Autodesk Inventor part; units mm, degrees
ref_plane "Work Plane3" through (-47.3429, 25.922, -109.9566) normal (0, 1, 0) x (1, 0, 0)
ref_plane "Work Plane4" through (-11.7245, 25.1265, -109.9566) normal (0, -1, 0) x (-1, 0, 0)
ref_plane "YZ Plane" through (0, 0, 0) normal (1, 0, 0) x (0, 1, 0)
sketch "Sketch1" plane through (0, 0, 0) normal (0, 0, 1) x (1, 0, 0)
  point P0 (0, 0)
sketch "Sketch2" plane through (0, 0, 0) normal (0, 1, 0) x (-1, 0, 0)
  line L0 (29.4419, 0) -> (29.4988, 0)
  arc A0 (58.9407, -29.4419) -> (29.4988, 0) centre (29.4988, -29.4419) ccw
  arc A1 (29.4419, 0) -> (0, -29.4419) centre (29.4419, -29.4419) ccw
  line L1 (0, -29.4419) -> (1.3334, -33.4091)
  line L2 (1.3334, -33.4091) -> (1.3334, -74.6587)
  line L3 (1.3334, -74.6587) -> (0, -77.6285)
  line L4 (0, -77.6285) -> (-1.0327, -97.9222)
  line L5 (58.9407, -29.4419) -> (57.7766, -33.4091)
  line L6 (57.7766, -33.4091) -> (57.7766, -76.7951)
  line L7 (57.7766, -76.7951) -> (58.9407, -78.9752)
  line L8 (58.9407, -78.9752) -> (59.9743, -95.7523)
  line L9 (59.9743, -95.7523) -> (60.0189, -96.4757)
  line L10 (-1.0327, -97.9222) -> (-0.9556, -96.5463)
  line L11 (11.7245, -109.9566) -> (47.3429, -109.9566)
  arc A2 (47.3429, -109.9566) -> (60.0189, -96.4757) centre (47.3429, -97.2566) ccw
  arc A3 (-0.9556, -96.5463) -> (11.7245, -109.9566) centre (11.7245, -97.2566) ccw
  point P0 (0, 0)
  point P1 (58.9407, 0)
  dimension "d5" = 29.4419
  dimension "d6" = 41.2496
  dimension "d7" = 20.32
  dimension "d8" = 12.7
extrude "Extrusion1" add sketch "Sketch2" along normal blind 29.5148
sketch "Sketch3" plane through (0, 29.5148, 0) normal (0, 1, 0) x (1, 0, 0)
  line L0 (-29.7463, 1.6533) -> (-29.8195, 1.6533)
  arc A0 (-58.3691, 30.2029) -> (-29.8195, 1.6533) centre (-29.8195, 30.2029) ccw
  arc A1 (-29.7463, 1.6533) -> (-1.1967, 30.2029) centre (-29.7463, 30.2029) ccw
  line L1 (-1.1967, 30.2029) -> (-2.4901, 33.4321)
  line L2 (-2.4901, 33.4321) -> (-2.4901, 73.4442)
  line L3 (-2.4901, 73.4442) -> (-0.5766, 76.9439)
  line L4 (-0.5766, 76.9439) -> (0.4251, 96.6289)
  line L5 (-58.3691, 30.2029) -> (-56.62, 33.4321)
  line L6 (-56.62, 33.4321) -> (-56.62, 75.5165)
  line L7 (-56.62, 75.5165) -> (-57.7491, 78.2503)
  line L8 (-57.7491, 78.2503) -> (-58.7517, 94.5241)
  line L9 (-58.7517, 94.5241) -> (-58.7949, 95.2257)
  line L10 (0.4251, 96.6289) -> (0.3503, 95.2942)
  line L11 (-11.9494, 108.3022) -> (-46.4992, 108.3022)
  arc A2 (-46.4992, 108.3022) -> (-58.7949, 95.2257) centre (-46.4992, 95.9832) ccw
  arc A3 (0.3503, 95.2942) -> (-11.9494, 108.3022) centre (-11.9494, 95.9832) ccw
  line L12 (-2.4901, 52.1447) -> (-2.4901, 53.4382) construction
  line L13 (-57.7766, 76.7951) -> (-57.7766, 33.4091) construction
  line L14 (-57.7766, 54.1324) -> (-56.62, 54.1324) construction
  arc A4 (-58.9407, 29.4419) -> (-29.4988, 0) centre (-29.4988, 29.4419) ccw construction
  line L15 (-29.4988, 0) -> (-29.4988, 1.6544) construction
  line L16 (-28.1015, 108.3022) -> (-28.1015, 109.9566) construction
  line L17 (-11.7245, 109.9566) -> (-47.3429, 109.9566) construction
  line L18 (-2.4901, 53.4382) -> (-1.3334, 53.4382) construction
  line L19 (-1.3334, 33.4091) -> (-1.3334, 74.6587) construction
  point P0 (0, 0)
  point P1 (-1.2057, 1.6533)
  point P2 (-58.3782, 1.6533)
  dimension "d9" = 28.5496
  dimension "d10" = 40.0121
  dimension "d11" = 19.7104
  dimension "d12" = 12.319
extrude "Extrusion2" cut sketch "Sketch3" against normal blind 25.4
sketch "Sketch4" plane through (0, 29.5148, 0) normal (0, 1, 0) x (1, 0, 0)
  point P0 (0, 0)
sketch "Sketch5" plane through (-11.7245, 0, -109.9566) normal (0, 0, -1) x (-1, 0, 0)
  line L0 (35.6184, 26.9603) -> (35.6184, 25.922)
  line L1 (35.6184, 0) -> (35.6184, 29.5148)
  line L2 (0, 0) -> (0, 29.5148)
  point P0 (-11.7245, 0)
sketch "Sketch6" plane through (0, 29.5148, 0) normal (0, 1, 0) x (1, 0, 0)
  point P0 (0, 0)
ref_plane "Work Plane3" through (-47.3429, 25.922, -109.9566) normal (0, 1, 0) x (1, 0, 0)
sketch "Sketch7" plane through (-47.3429, 25.922, -109.9566) normal (0, 1, 0) x (1, 0, 0)
  line L0 (46.0094, -76.5475) -> (46.0094, -35.2979)
  line L1 (46.0094, -35.2979) -> (47.3429, -32.3281)
  line L2 (47.3429, -32.3281) -> (48.2985, -13.4103)
  line L3 (48.2985, -13.4103) -> (48.3756, -12.0344)
  line L4 (46.0094, -76.5475) -> (47.3429, -80.5147)
  line L5 (0, 0) -> (35.6184, 0)
  line L6 (-12.676, -13.4809) -> (-11.5978, -30.9814)
  line L7 (-11.5978, -30.9814) -> (-10.4337, -33.1615)
  line L8 (-10.4337, -33.1615) -> (-10.4337, -76.5475)
  line L9 (-10.4337, -76.5475) -> (-11.5978, -80.5147)
  arc A0 (-11.5978, -80.5147) -> (47.3429, -80.5147) centre (17.8725, -80.5147) ccw
  arc A1 (48.3756, -12.0344) -> (35.6184, 0) centre (35.6184, -12.7789) ccw
  line L10 (-12.676, -13.4809) -> (-11.5978, -30.9814)
  arc A2 (0, 0) -> (-12.676, -13.4809) centre (0, -12.7) ccw
  line L11 (46.0094, -76.5475) -> (46.0094, -35.2979)
  line L12 (46.0094, -35.2979) -> (47.3429, -32.3281)
  line L13 (47.3429, -32.3281) -> (48.2985, -13.4103)
  line L14 (48.2985, -13.4103) -> (48.3756, -12.0344)
  line L15 (46.0094, -76.5475) -> (47.3429, -80.5147)
  line L16 (0, 0) -> (35.6184, 0)
  line L17 (-12.676, -13.4809) -> (-11.5978, -30.9814)
  line L18 (-11.5978, -30.9814) -> (-10.4337, -33.1615)
  line L19 (-10.4337, -33.1615) -> (-10.4337, -76.5475)
  line L20 (-10.4337, -76.5475) -> (-11.5978, -80.5147)
  arc A3 (-11.5978, -80.5147) -> (47.3429, -80.5147) centre (17.8725, -80.5147) ccw
  arc A4 (48.3756, -12.0344) -> (35.6184, 0) centre (35.6184, -12.7789) ccw
  arc A5 (0, 0) -> (-12.676, -13.4809) centre (0, -12.7) ccw
  point P0 (47.3429, -109.9566)
sketch "Sketch8" plane through (-11.7245, 0, -109.9566) normal (0, 0, -1) x (-1, 0, 0)
  line L0 (0, 0) -> (0, 29.5148)
  line L1 (0, 25.1265) -> (35.5035, 25.1265)
  point P0 (-11.7245, 0)
ref_plane "Work Plane4" through (-11.7245, 25.1265, -109.9566) normal (0, -1, 0) x (-1, 0, 0)
sketch "Sketch9" plane through (-11.7245, 25.1265, -109.9566) normal (0, -1, 0) x (-1, 0, 0)
  line L0 (0, 0) -> (35.6184, 0)
  line L1 (46.0521, -76.5475) -> (47.2162, -80.5147)
  line L2 (48.2944, -13.4809) -> (47.2162, -31.0011)
  line L3 (47.2162, -31.0011) -> (46.0521, -33.1615)
  line L4 (46.0521, -33.1615) -> (46.0521, -76.5475)
  line L5 (-12.6801, -13.4103) -> (-12.7572, -12.0344)
  line L6 (-12.6801, -13.4103) -> (-11.7245, -32.3281)
  line L7 (-11.7245, -32.3281) -> (-10.3911, -35.2979)
  line L8 (-10.3911, -35.2979) -> (-10.3911, -76.5475)
  line L9 (-10.3911, -76.5475) -> (-11.7245, -80.5147)
  arc A0 (-11.7245, -80.5147) -> (47.2162, -80.5147) centre (17.7459, -80.4862) ccw
  arc A1 (0, 0) -> (-12.7572, -12.0344) centre (0, -12.7789) ccw
  arc A2 (48.2944, -13.4809) -> (35.6184, 0) centre (35.6184, -12.7) ccw
  point P0 (-11.7245, -109.9566)
  point P1 (17.7174, -109.9566)
properties part number "Random Object"
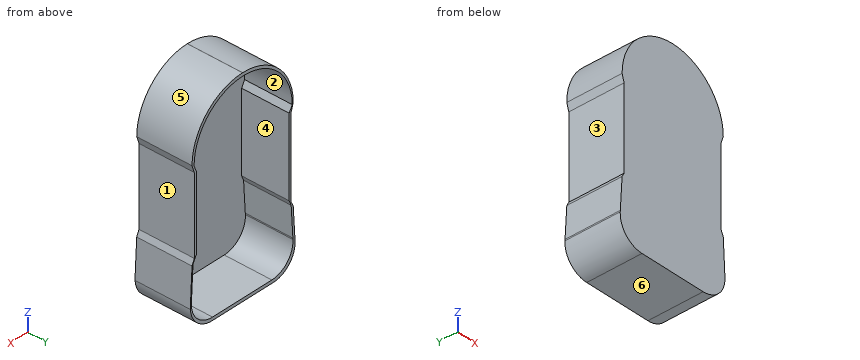
Check sheet for the modelled part. Datum: model origin and axes. Units: mm. Face numbers are marked on the shaded views. A direction names the side the tool comes from. Give positions to 0.01 mm unless a question says otherwise; leave off trailing zeros. Loops run counter-clockwise (first coordinate to the right, second up) from the corner with the lowest first, then second, coordinate; pieces in that order, holes last. Notation, with made-up numbers: M 33,82.5 L 83,82.5 A16 ccw 83,112.5 Z; hole C 1.5,24 d5. An arc over 180 degrees is marked long. Answer in a Markdown table with one row per item.
1) Mould release check, pull along Z, two halves, no side actions. Record for the marked faces 4, 5 and 6: released by +Z, released by -Z, zero draft, split by the parting line, or undercut.
Solutions:
| item | result |
|---|---|
| face 4 | undercut |
| face 5 | released by +Z |
| face 6 | released by -Z |
2) Tool access check on the marked faces 1, 2 and 3. Record the directions out of +Z, -Z, +X, -X, +Y, -Y that give a thin tool (end or side, any length) a straight path to the whole face; none if there is none.
Solutions:
| item | result |
|---|---|
| face 1 | +X, +Y, -Y |
| face 2 | +Y |
| face 3 | -X, +Y, -Y |
3) Cross-section at C-C (z = -38). Enter the section's corners in (x, y).
Solutions:
| item | result |
|---|---|
| outline | M -57.78,0 L -1.33,0 L -1.33,29.51 L -2.49,29.51 L -2.49,4.11 L -56.62,4.11 L -56.62,29.51 L -57.78,29.51 Z |
4) Cross-section at B-B (x = -9.5). Enter the section's corners in (y, z), plus the area to 3 significant figures.
Solutions:
| item | result |
|---|---|
| outline | M 0,-109.76 L 29.51,-109.76 L 29.51,-108.06 L 4.11,-108.06 L 4.11,-10.07 L 29.51,-10.07 L 29.51,-7.78 L 0,-7.78 Z |
| area | 521 mm^2 |
5) Thickness scan on line 1 (X direction, y = 4.75, z = -73); line 2 (Z direction, x = -29, y = 26.75); line 3 (Y direction, x = -29.5, z = -52). Record the ranges inside material, lowest first.
Solutions:
| item | result |
|---|---|
| line 1 | x = -57.78 to -56.62, -2.49 to -1.33 |
| line 2 | z = -109.96 to -108.3, -1.66 to 0 |
| line 3 | y = 0 to 4.11 |
6) Depth check by flat-ended pin: pin 1 (7.5 mm diameter, centred on x = -36.5, y = 20, fed in from +Z); pin 2 (6 mm diameter, centred on x = -42.5, z = -89.5, fed in from +Y); pin 3 (4 mm diameter, centred on x = -9.5, y = 23.5, fed in from +Z); pin 4 (6 mm diameter, centred on x = -25, z = -46.5, fed in from -Y). Enter the tip coordinate at first touch or a pass-through.
Solutions:
| item | result |
|---|---|
| pin 1 | stops at z = -0.18 |
| pin 2 | stops at y = 4.11 |
| pin 3 | stops at z = -6.1 |
| pin 4 | stops at y = 0 |
